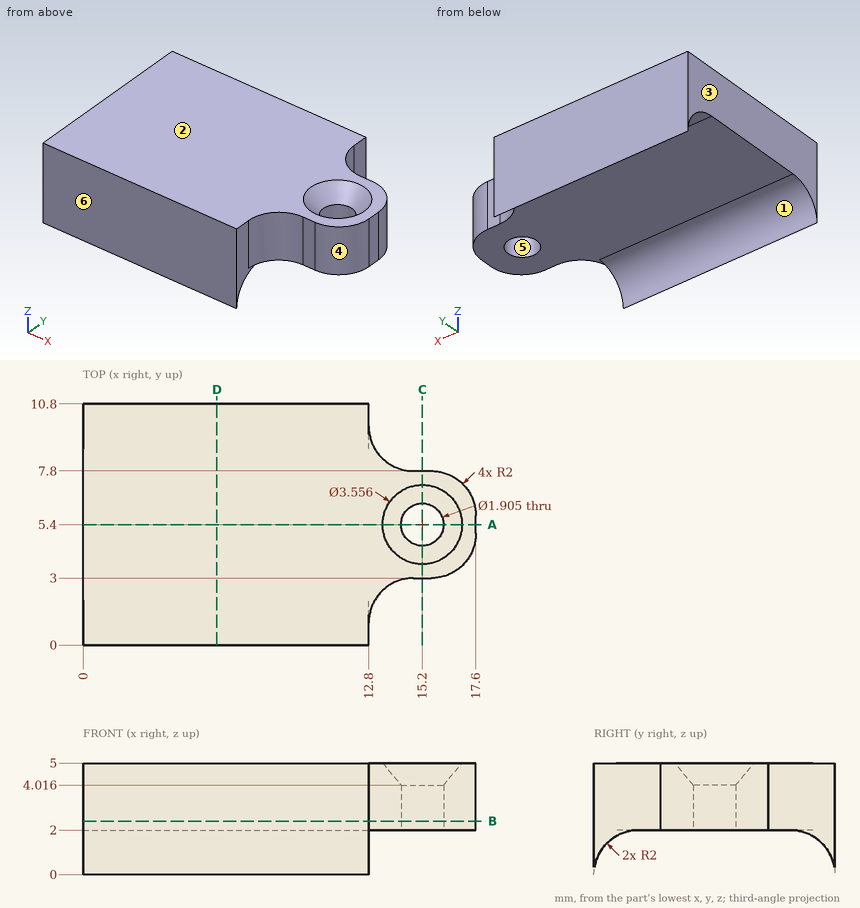
Design review of the part shown in the three views and the two pictorial views. Dimensions are in mm from the part's minimum x, y and z. A direction names the side the tool comes from. Give positions to 0.01 mm unless a question says otherwise; leave off trailing zeros. Loops run counter-clockwise (first coordinate to the right, second up) from the corner with the lowest first, then second, coordinate; pieces in that order, holes last. Notation, with made-up numbers: (80.5, -13) -> (132.5, -13) arc R10 ccw to (132.5, 4) -> close; hole circle Ø8 at (56.25, 49.25). An arc over 180 degrees is marked (long way). One line per question, with ' | ' between items.
1) We need section A-A (y = 5.4). Write out the cut boundary in (x, z).
Resolved:
outline: (0, 2) -> (14.25, 2) -> (14.25, 4.02) -> (13.42, 5) -> (0, 5) -> close; (16.15, 2) -> (17.6, 2) -> (17.6, 5) -> (16.98, 5) -> (16.15, 4.02) -> close
2) We need section D-D (x = 6). Write out the cut boundary in (y, z).
Resolved:
outline: (0, 0) arc R2 cw to (2, 2) -> (8.8, 2) arc R2 cw to (10.8, 0) -> (10.8, 5) -> (0, 5) -> close
3) Insertion check: pin 1 Ø1.6 at (y, z) = (0.5, 2.5) entering from +X; pin 2 Ø2 at (y, z) = (9.5, 1.5) entering from +X (1 decimal); pin 3 Ø4 at (x, y) = (14.5, 5) entering from -Z; pin 4 Ø1.1 at (x, y) = (15.2, 5.4) entering from -Z. Each pin has a flat end and moves straight along its axis. Give the tip position at first contact, or say it passes through.
Resolved:
pin 1: stops at x = 12.82 | pin 2: stops at x = 13.2 | pin 3: stops at z = 2 | pin 4: passes through
4) The part is to be moulded in two halves that separate along X. For the marked faces 3, 4, 5 and 6, say which applies: +X half, -X half, draft (parallel to the pull), parting line (faces both ways), or undercut.
Resolved:
face 3: -X half | face 4: +X half | face 5: undercut | face 6: draft
5) To check wall thickness, follow probe 1 along Y at (x, z) = (15.2, 3.55); probe 2 along X at (y, z) = (5.4, 3.5); probe 3 along Z at (x, y) = (12.25, 2.75). State the ranges of each line that lie inside material, in increasing order.
Resolved:
probe 1: y = 3 to 4.45, 6.35 to 7.8 | probe 2: x = 0 to 14.25, 16.15 to 17.6 | probe 3: z = 2 to 5
6) For the marked faces 1 and 2, list the 3-axis set-ups (+Z, -Z, +X, -X, +Y, -Y) from which the entire face can be reached by the end or side of a thin tool; tool diameter is ignored.
Resolved:
face 1: -Z, +X, -X | face 2: +Z, +X, -X, +Y, -Y
7) We need section B-B (z = 2.4). Write out the cut boundary in (x, y) (1 decimal), plus the area to 3 significant figures.
Resolved:
outline: (0, 0) -> (12.8, 0) -> (12.8, 1) arc R2 cw to (14.8, 3) -> (15.6, 3) arc R2 ccw to (17.6, 5) -> (17.6, 5.8) arc R2 ccw to (15.6, 7.8) -> (14.8, 7.8) arc R2 cw to (12.8, 9.8) -> (12.8, 10.8) -> (0, 10.8) -> close; hole circle Ø1.9 at (15.2, 5.4) | area: 158 mm2
8) We need section C-C (x = 15.2). Write out the cut boundary in (y, z).
Resolved:
outline: (3, 2) -> (4.45, 2) -> (4.45, 4.02) -> (3.62, 5) -> (3, 5) -> close; (6.35, 2) -> (7.8, 2) -> (7.8, 5) -> (7.18, 5) -> (6.35, 4.02) -> close
